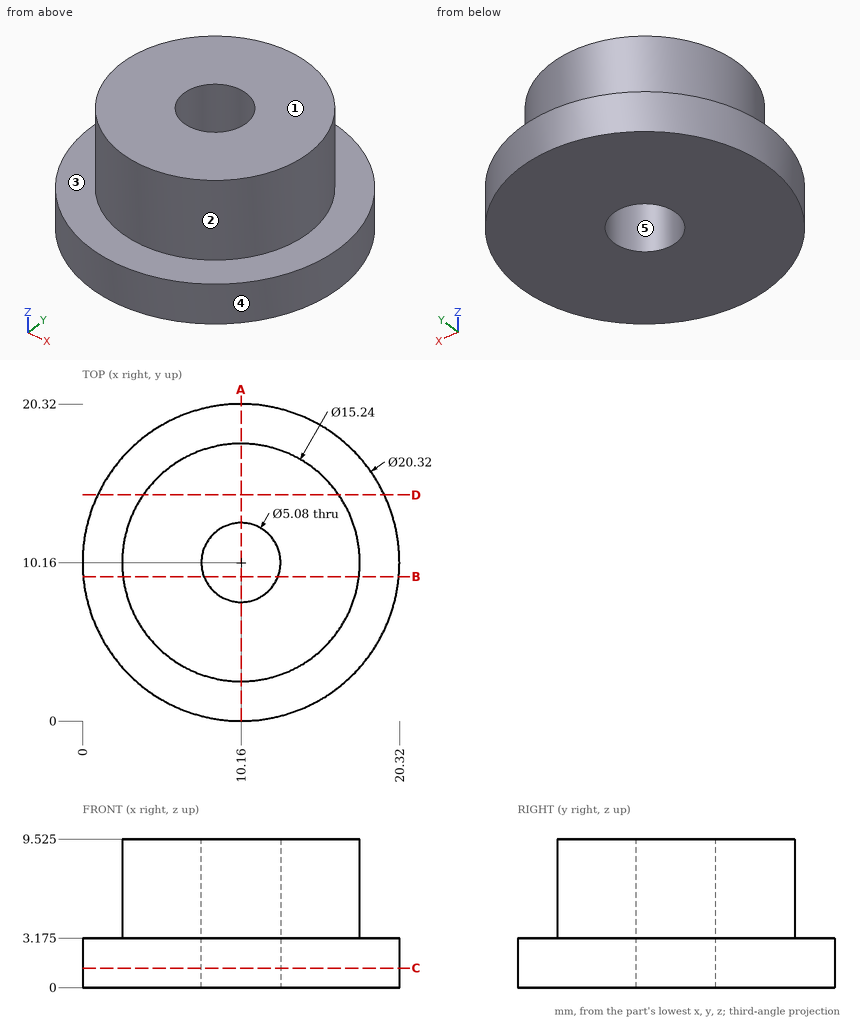
Could you check a few things on this drawing? It's one solid part, dimensions in mm from its lowest x, y, z. A direction names the side the tool comes from. Coordinates: 2 decimals unless noted, no trailing zeros. Order: outer loops, then holes, each group sorted by start corner. A loop starts at its lowest first (then second) coordinate and runs counter-clockwise, first axis right, second up. Notation, with made-up numbers: (77.25, 76) - (115.25, 76) arc R19 cw to (115.25, 92) - close; hole circle Ø11 at (83, 76). An arc over 180 degrees is marked (long way). Answer as a JSON object with one key per item and string values. Group by question number.
Q1. Will these pins go through, and if not, where does the flat tip stop? P1, Ø2, axis at x = 8.5, z = 8, coming from the -Y side; P2, Ø1.5, axis at y = 16.5, z = 5.5, coming from the -X side; P3, Ø1, axis at x = 10.5, z = 8, coming from the -Y side; P4, Ø6, axis at x = 10.16, y = 10.16, coming from the +Z side (3 decimals).
Q2. Imagine slicing it at C-C (z = 1.25). Please give me the cut outline in (x, y).
Q3. I need wall thicknesses on line 1 (Y direction, x = 10.16, z = 5); line 2 (Y direction, x = 10.16, z = 2.5); line 3 (Z direction, x = 17, y = 15) (3 decimals). Which ranges of each line are inside material? Lowest first, please. Write a range as from..to.
Q4. Imagine slicing it at B-B (y = 9.25). Please give me the cut outline in (x, z) (3 decimals), and give its area (3 significant figures).
Q5. Imagine slicing it at A-A (x = 10.16). Please give me the cut outline in (y, z) (3 decimals), and give its area (3 significant figures).
Q6. Imagine slicing it at D-D (y = 14.5). Please give me the cut outline in (x, z) (3 decimals).
Q7. We'd pull the mould along X, two halves only. Please class the marked faces 3, 4 and 5: +X half, -X half, draft (parallel to the pull), parting line (faces both ways), or undercut.
Q8. On a 3-axis mill with a long thin cutter (end or side, diameter ignored), from which of +Z, -Z, +X, -X, +Y, -Y can I reach the whole of each face in a straight line? I mean the marked faces 1 and 2. Say none if no direction works.
Determined:
{
 "1": {"P1": "stops at y = 2.57", "P2": "stops at x = 4.98", "P3": "stops at y = 2.54", "P4": "stops at z = 9.525"},
 "2": {"outline": "circle Ø20.32 at (10.16, 10.16); hole circle Ø5.08 at (10.16, 10.16)"},
 "3": {"line 1": "y = 2.54..7.62, 12.7..17.78", "line 2": "y = 0..7.62, 12.7..20.32", "line 3": "z = 0..3.175"},
 "4": {"outline": "(0.041, 0) - (7.789, 0) - (7.789, 9.525) - (2.595, 9.525) - (2.595, 3.175) - (0.041, 3.175) - close; (12.531, 0) - (20.279, 0) - (20.279, 3.175) - (17.725, 3.175) - (17.725, 9.525) - (12.531, 9.525) - close", "area": "115 mm2"},
 "5": {"outline": "(0, 0) - (7.62, 0) - (7.62, 9.525) - (2.54, 9.525) - (2.54, 3.175) - (0, 3.175) - close; (12.7, 0) - (20.32, 0) - (20.32, 3.175) - (17.78, 3.175) - (17.78, 9.525) - (12.7, 9.525) - close", "area": "113 mm2"},
 "6": {"outline": "(0.974, 0) - (19.346, 0) - (19.346, 3.175) - (16.423, 3.175) - (16.423, 9.525) - (3.897, 9.525) - (3.897, 3.175) - (0.974, 3.175) - close"},
 "7": {"face 3": "draft", "face 4": "parting line", "face 5": "undercut"},
 "8": {"face 1": "+Z, +X, -X, +Y, -Y", "face 2": "+Z"}
}
